Could you check a few things on this model? Use its own coordinates, in mm. Face numbers are marked on the shaded views. Give positions to 0.01 mm unless a question says otherwise; leave off trailing zeros. Loops run counter-clockwise (first coordinate to the right, second up) from the corner with the lowest first, then second, coordinate; pieces in that order, holes last. Notation, with made-up numbers: M 27,63 L 49,63 A21 ccw 49,79 Z; hole C 31,-33 d7. An arc over 180 degrees is marked long. Use a Markdown table: item, result. Add a question column.
1) Suppose I cut it at D-D on z = -1.7. List the corners of the cut face in (x, y) for me, and give its area (3 significant figures).
2) Suppose I cut it at A-A on z = 0. List the corners of the cut face in (x, y) for me.
3) We'd pull the mould along Z, two halves only. Please class the marked faces 1, 2, 3 and 4: +Z half, -Z half, draft (parallel to the pull), parting line (faces both ways), or undercut.
4) Suppose I cut it at B-B on y = 0.8. List the corners of the cut face in (x, z) for me, and give its area (3 significant figures).
5) Suppose I cut it at C-C on x = -7.75. List the corners of the cut face in (y, z) for me, and give its area (3 significant figures).
6) Will these pins go through, and if not, where does the flat tip stop? pin 1 Ø1.1 at (x, z) = (1, 0) entering from +Y; pin 2 Ø3 at (x, y) = (-3.5, -1.5) entering from -Z; pin 3 Ø1.5 at (x, z) = (-7.5, 2) entering from +Y.
7) If I drill on line 1 along X through (y, z) = (-0.5, -0.7); line 2 along Y through (x, z) = (-10.25, 0.05); line 3 along Z through (x, y) = (-0.75, -0.75), over which ranges is the centre line in solid material (lowest first)? Write a range as [from, to].
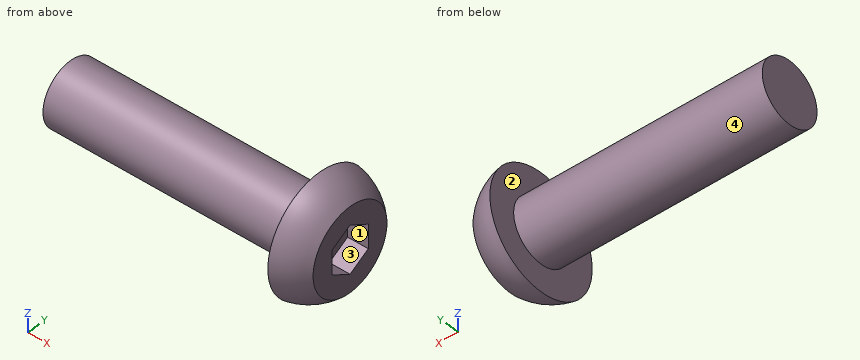
Autodesk Inventor part; units mm, degrees
ref_plane "YZ Plane" through (0, 0, 0) normal (1, 0, 0) x (0, 1, 0)
ref_plane "XZ Plane" through (0, 0, 0) normal (0, 1, 0) x (-1, 0, 0)
ref_plane "XY Plane" through (0, 0, 0) normal (0, 0, 1) x (1, 0, 0)
sketch "Sketch1" plane through (0, 0, 0) normal (0, 0, 1) x (1, 0, 0)
  line L0 (0, 0) -> (-12, 0)
  line L1 (-12, 0) -> (-12, 1.5)
  line L2 (-12, 1.5) -> (0, 1.5)
  line L3 (0, 1.5) -> (0, 0)
  line L4 (0, 0) -> (1.5, 0)
  line L5 (1.5, 0) -> (1.5, 2.8)
  line L6 (1.5, 2.8) -> (0, 2.8)
  line L7 (0, 2.8) -> (0, 0)
  circle A0 centre (-0.5, 0) radius 2.8443
  point P0 (1.5, 2.0224)
  dimension "d0" = 12
  dimension "d1" = 1.5
  dimension "d2" = 2.8
  dimension "d3" = 1.5
  dimension "d4" = 0.5
revolve "Revolution1" add sketch "Sketch1" angle 360 about axis through (0, 0, 0) along (-1, 0, 0) contours L0 A0 L2 L3 | L3 L7 A0 L5 L4 | L0 L1 L2 A0
thread "Thread1"
sketch "Sketch2" plane through (1.5, 0, 0) normal (1, 0, 0) x (0, 0, -1)
  line L0 (0.5774, 1) -> (1.1547, 0)
  line L1 (1.1547, 0) -> (0.5774, -1)
  line L2 (0.5774, -1) -> (-0.5774, -1)
  line L3 (-0.5774, -1) -> (-1.1547, 0)
  line L4 (-1.1547, 0) -> (-0.5774, 1)
  line L5 (-0.5774, 1) -> (0.5774, 1)
  point P0 (0, 0)
  point P1 (0, 0)
  point P2 (0, -1)
  dimension "d8" = 2
extrude "Extrusion1" cut sketch "Sketch2" against normal blind 1
properties part number "M3 x 12 Button"
Answer block:
| question | item | result |
|---|---|---|
| 1 | outline | M 0,-2.22 A2.28 ccw 1.5,-1.1 L 1.5,1.1 A2.28 ccw 0,2.22 Z |
| 1 | area | 5.49 mm^2 |
| 2 | outline | M -12,-1.5 L 0,-1.5 L 0,-2.8 A2.84 ccw 1.5,-2.02 L 1.5,-1 L 0.5,-1 L 0.5,1 L 1.5,1 L 1.5,2.02 A2.84 ccw 0,2.8 L 0,1.5 L -12,1.5 Z |
| 3 | face 1 | undercut |
| 3 | face 2 | draft |
| 3 | face 3 | undercut |
| 3 | face 4 | parting line |
| 4 | outline | M -12,-1.27 L 0,-1.27 L 0,-2.68 A2.73 ccw 1.5,-1.86 L 1.5,-0.69 L 0.5,-0.69 L 0.5,0.69 L 1.5,0.69 L 1.5,1.86 A2.73 ccw 0,2.68 L 0,1.27 L -12,1.27 Z |
| 4 | area | 36.2 mm^2 |
| 5 | outline | C 0,0 d3 |
| 5 | area | 7.07 mm^2 |
| 6 | pin 1 | stops at y = 2.68 |
| 6 | pin 2 | stops at z = -1.5 |
| 6 | pin 3 | stops at y = 0.83 |
| 7 | line 1 | x = [-12, 0.5] |
| 7 | line 2 | y = [-1.5, 1.5] |
| 7 | line 3 | z = [-1.3, 1.3] |
